from build123d import *

# Parameters (mm, degrees)
SKETCH1_W           = 40
SKETCH1_H           = 18
BOSS_EXTRUDE1_DEPTH = 18.47
CUT_EXTRUDE1_REACH  = 20
SKETCH2_R           = 10.5
CUT_EXTRUDE3_REACH  = 42
SKETCH4_R           = 6
CUT_EXTRUDE4_REACH  = 20.47
SKETCH5_W           = 5
SKETCH5_H           = 18
SKETCH6_W           = 40
SKETCH6_H           = 40
BOSS_EXTRUDE2_DEPTH = 10
CUT_EXTRUDE5_REACH  = 12
SKETCH7_R           = 2


with BuildPart() as part:
    # Sketch1 → Boss-Extrude1 (new body)
    with BuildSketch(Plane(origin=(0, 0, 0), x_dir=(1, 0, 0), z_dir=(0, 1, 0))):
        Rectangle(SKETCH1_W, SKETCH1_H)
    extrude(amount=BOSS_EXTRUDE1_DEPTH)

    # Sketch2 → Cut-Extrude1 (cut, up to next)
    with BuildSketch(Plane.XY.offset(9), mode=Mode.PRIVATE) as cut_extrude1_sk1:
        Circle(SKETCH2_R)
    cut_extrude1_tool1 = extrude(cut_extrude1_sk1.sketch, amount=-CUT_EXTRUDE1_REACH, mode=Mode.PRIVATE) & part.part
    add(cut_extrude1_tool1.solids().sort_by_distance((0, 0, 9))[0], mode=Mode.SUBTRACT)

    # Sketch4 → Cut-Extrude3 (cut, up to next)
    with BuildSketch(Plane.ZY.offset(20), mode=Mode.PRIVATE) as cut_extrude3_sk1:
        Circle(SKETCH4_R)
    cut_extrude3_tool1 = extrude(cut_extrude3_sk1.sketch, amount=-CUT_EXTRUDE3_REACH, mode=Mode.PRIVATE) & part.part
    add(cut_extrude3_tool1.solids().sort_by_distance((-20, 0, 0))[0], mode=Mode.SUBTRACT)

    # Sketch5 → Cut-Extrude4 (cut, up to next)
    with BuildSketch(Plane.XZ, mode=Mode.PRIVATE) as cut_extrude4_sk1:
        with Locations((-17.5, 0)):
            Rectangle(SKETCH5_W, SKETCH5_H)
    cut_extrude4_tool1 = extrude(cut_extrude4_sk1.sketch, amount=-CUT_EXTRUDE4_REACH, mode=Mode.PRIVATE) & part.part
    add(cut_extrude4_tool1.solids().sort_by_distance((-17.5, 0, 0))[0], mode=Mode.SUBTRACT)

    # Sketch6 → Boss-Extrude2 (add)
    with BuildSketch(Plane(origin=(0, 18.47, 0), x_dir=(1, 0, 0), z_dir=(0, 1, 0))):
        Rectangle(SKETCH6_W, SKETCH6_H)
    extrude(amount=BOSS_EXTRUDE2_DEPTH)

    # Sketch7 → Cut-Extrude5 (cut, up to next)
    with BuildSketch(Plane.XZ.offset(-18.47), mode=Mode.PRIVATE) as cut_extrude5_sk1:
        with Locations((16, 16)):
            Circle(SKETCH7_R)
    cut_extrude5_tool1 = extrude(cut_extrude5_sk1.sketch, amount=-CUT_EXTRUDE5_REACH, mode=Mode.PRIVATE) & part.part
    add(cut_extrude5_tool1.solids().sort_by_distance((16, 18.47, 16))[0], mode=Mode.SUBTRACT)
    # Sketch7 → Cut-Extrude5 (cut, up to next)
    with BuildSketch(Plane.XZ.offset(-18.47), mode=Mode.PRIVATE) as cut_extrude5_sk2:
        with Locations((-16, 16)):
            Circle(SKETCH7_R)
    cut_extrude5_tool2 = extrude(cut_extrude5_sk2.sketch, amount=-CUT_EXTRUDE5_REACH, mode=Mode.PRIVATE) & part.part
    add(cut_extrude5_tool2.solids().sort_by_distance((-16, 18.47, 16))[0], mode=Mode.SUBTRACT)
    # Sketch7 → Cut-Extrude5 (cut, up to next)
    with BuildSketch(Plane.XZ.offset(-18.47), mode=Mode.PRIVATE) as cut_extrude5_sk3:
        with Locations((16, -16)):
            Circle(SKETCH7_R)
    cut_extrude5_tool3 = extrude(cut_extrude5_sk3.sketch, amount=-CUT_EXTRUDE5_REACH, mode=Mode.PRIVATE) & part.part
    add(cut_extrude5_tool3.solids().sort_by_distance((16, 18.47, -16))[0], mode=Mode.SUBTRACT)
    # Sketch7 → Cut-Extrude5 (cut, up to next)
    with BuildSketch(Plane.XZ.offset(-18.47), mode=Mode.PRIVATE) as cut_extrude5_sk4:
        with Locations((-16, -16)):
            Circle(SKETCH7_R)
    cut_extrude5_tool4 = extrude(cut_extrude5_sk4.sketch, amount=-CUT_EXTRUDE5_REACH, mode=Mode.PRIVATE) & part.part
    add(cut_extrude5_tool4.solids().sort_by_distance((-16, 18.47, -16))[0], mode=Mode.SUBTRACT)


solid = part.part
The listing builds one solid part. Answer for the finished solid, in the listing's coordinates (mm). A direction names the side the tool comes from. Coordinates: 2 decimals unless noted, no trailing zeros. Write each loop counter-clockwise with the first axis right and the second up, starting at its lowest first coordinate (ties: lowest second). Pieces come first, ordered by that corner, then holes. Notation, with made-up numbers: M 73.5,44.5 L 105.5,44.5 A24 cw 105.5,67.5 Z; hole C 29,60.5 d3. An arc over 180 degrees is marked long. Write each question's results on one line, items separated by ' | '.
Item 1: The part is cut by section B-B on y = 20.25. Determine the outline of the cut face in (x, z).
Answer below:
outline: M -20,-20 L 20,-20 L 20,20 L -20,20 Z; hole C -16,-16 d4; hole C -16,16 d4; hole C 16,-16 d4; hole C 16,16 d4
Item 2: For a pull along Z with two mould halves and no side action, classify faces 4 (the face through (-16, 23, 18)), 5 (the face through (-20, 23, 0)), 6 (the face through (2, 11, 9)), 7 (the face through (2, 11, -9)) as released by +Z, released by -Z, zero draft, split by the parting line, or undercut.
Answer below:
face 4: undercut | face 5: zero draft | face 6: released by +Z | face 7: released by -Z
Item 3: Which of the six approach directions +Z, -Z, +X, -X, +Y, -Y give full straight-line access (tool end or side, diameter ignored) to faces 1 (the face through (-13, 6, 0)), 2 (the face through (-15, 11, 0)), 3 (the face through (-13, 0, -8))?
Answer below:
face 1: -X, -Y | face 2: +Z, -Z, -X, -Y | face 3: +Z, -Z, +X, -X, -Y
Item 4: The part is cut by section C-C on z = 7. Determine the outline of the cut face in (x, y).
Answer below:
outline: M -20,18.47 L -15,18.47 L -15,0 L -10.5,0 A10.5 cw 10.5,0 L 20,0 L 20,28.47 L -20,28.47 Z
Item 5: Consider probe 1 along Z at (x, y) = (16, 26); probe 2 along X at (y, z) = (20.5, -14.5); probe 3 along Y at (x, z) = (4, -15). Determine where each line is inside the solid, lowest interval first. Write a range as [from, to].
Answer below:
probe 1: [-20, -18], [-14, 14], [18, 20] | probe 2: [-20, -17.32], [-14.68, 14.68], [17.32, 20] | probe 3: [18.47, 28.47]
Item 6: The part is cut by section D-D on y = 7.5. Determine the outline of the cut face in (x, z).
Answer below:
outline: M -15,-9 L -7.35,-9 L -7.35,9 L -15,9 Z; M 7.35,-9 L 20,-9 L 20,9 L 7.35,9 Z
Item 7: Given P1, Ø8, axis at x = 4.5, z = -1.5, coming from the -Y side; P2, Ø1.5, axis at x = 8, z = -3, coming from the -Y side; P3, Ø2, axis at x = 6, z = 2, coming from the -Y side; P4, Ø6.5, axis at x = 16, z = -16, coming from the +Y side, each flat-ended and moving along its own axis, determine where each tip first touches the part or whether it passes through.
Answer below:
P1: y = 6.16 | P2: y = 5.8 | P3: y = 7.83 | P4: y = 28.47
Item 8: The part is cut by section A-A on x = 16. Determine the outline of the cut face in (y, z), and give its area (3 significant figures).
Answer below:
outline: M 0,-9 L 18.47,-9 L 18.47,-14 L 28.47,-14 L 28.47,14 L 18.47,14 L 18.47,9 L 0,9 Z; M 18.47,-20 L 28.47,-20 L 28.47,-18 L 18.47,-18 Z; M 18.47,18 L 28.47,18 L 28.47,20 L 18.47,20 Z | area: 652 mm2
